Here's how the part is built. I have some questions about the finished solid (model axes, mm). A direction names the side the tool comes from. Give positions to 0.01 mm unless a question says otherwise; leave off trailing zeros. Loops run counter-clockwise (first coordinate to the right, second up) from the corner with the lowest first, then second, coordinate; pieces in that order, holes last. Notation, with made-up numbers: (78.5, 72.5) - (89.5, 72.5) arc R19 cw to (89.5, 105.5) - close; hole circle Ø5 at (20, 84.25). An arc over 180 degrees is marked (long way). Use one line per item in the form item = value.
from build123d import *

# Parameters (mm, degrees)
EXTRUDE_1_DEPTH           = 200
CUT_EXTRUDE_START         = -130
CUT_EXTRUDE_1_OUTLINE_W   = 315
CUT_EXTRUDE_1_OUTLINE_H   = 262
CUT_EXTRUDE_1_DEPTH       = 65
CUT_EXTRUDE_START_2       = 65
CUT_EXTRUDE_1_2_OUTLINE_W = 315
CUT_EXTRUDE_1_2_OUTLINE_H = 262
CUT_EXTRUDE_1_2_DEPTH     = 65
SHELL_START               = 5
SHELL_1_OUTLINE_W         = 125
SHELL_1_OUTLINE_H         = 250
SHELL_1_DEPTH             = 190
EXTRUDE_7_DEPTH           = 3
SKETCH_5_R                = 5
EXTRUDE_8_DEPTH           = 5
SKETCH_6_R                = 38
SKETCH_6_R_2              = 16
EXTRUDE_9_DEPTH           = 15
SKETCH_7_R                = 10
SKETCH_7_R_2              = 5
EXTRUDE_10_DEPTH          = 15
SKETCH_8_R                = 1.5
CUT_EXTRUDE_2_DEPTH       = 10


with BuildPart() as part:
    # 草图1 → 旋转1 (revolve)
    with BuildSketch(Plane.XY):
        with BuildLine():
            Line((0, 130), (0, -130))
            ThreePointArc((0, -130), (130, 0), (0, 130))
        make_face()
    revolve(axis=Axis((0, 130, 0), (0, -1, 0)))

    # 草图3 → 凸台-拉伸1 (add)
    with BuildSketch(Plane(origin=(0, 0, 0), x_dir=(1, 0, 0), z_dir=(0, 1, 0))):
        with BuildLine():
            Line((-120, -130), (120, -130))
            ThreePointArc((120, -130), (127.071067812, -127.071067812), (130, -120))
            Line((130, -120), (130, 120))
            ThreePointArc((130, 120), (127.071067812, 127.071067812), (120, 130))
            Line((120, 130), (-120, 130))
            ThreePointArc((-120, 130), (-127.071067812, 127.071067812), (-130, 120))
            Line((-130, 120), (-130, -120))
            ThreePointArc((-130, -120), (-127.071067812, -127.071067812), (-120, -130))
        make_face()
    extrude(amount=EXTRUDE_1_DEPTH)

    # 切除-拉伸1: read off the stored shape, not the designer's step
    # 切除-拉伸1 outline → 切除-拉伸1 (cut)
    with BuildSketch(Plane.YZ.offset(CUT_EXTRUDE_START)):
        with Locations((43.5, 0)):
            Rectangle(CUT_EXTRUDE_1_OUTLINE_W, CUT_EXTRUDE_1_OUTLINE_H)
    extrude(amount=CUT_EXTRUDE_1_DEPTH, mode=Mode.SUBTRACT)

    # Cut-Extrude 1 2 outline → Cut-Extrude 1 2 (cut)
    with BuildSketch(Plane.YZ.offset(CUT_EXTRUDE_START_2)):
        with Locations((43.5, 0)):
            Rectangle(CUT_EXTRUDE_1_2_OUTLINE_W, CUT_EXTRUDE_1_2_OUTLINE_H)
    extrude(amount=CUT_EXTRUDE_1_2_DEPTH, mode=Mode.SUBTRACT)

    # 抽壳1: read off the stored shape, not the designer's step
    # 抽壳1 outline → 抽壳1 (cut)
    with BuildSketch(Plane(origin=(0, 0, 0), x_dir=(1, 0, 0), z_dir=(0, 1, 0)).offset(SHELL_START)):
        with Locations((-2.5, 0)):
            Rectangle(SHELL_1_OUTLINE_W, SHELL_1_OUTLINE_H)
    extrude(amount=SHELL_1_DEPTH, mode=Mode.SUBTRACT)

    # Shell 1 2 outline → Shell 1 2 (revolve, cut)
    with BuildSketch(Plane.YX):
        with BuildLine():
            Line((109.658560943, 60.0000001), (0, 60.000000075))
            Line((0, 60.000000075), (0, -65.0000001))
            Line((0, -65.0000001), (106.770782459, -65.0000001))
            ThreePointArc((106.770782459, -65.0000001), (124.966656288, -2.887008165), (109.658560943, 60.0000001))
        make_face()
    revolve(axis=Axis((0, 0, 0), (1, 0, 0)), mode=Mode.SUBTRACT)

    # 草图4 → 凸台-拉伸7 (add)
    with BuildSketch(Plane.ZY.offset(65)):
        with BuildLine():
            Line((-130, 135), (-130, 0))
            Line((-130, 0), (-112.249721603, 0))
            ThreePointArc((-112.249721603, 0), (0, 112.249721603), (112.249721603, 0))
            Line((112.249721603, 0), (130, 0))
            Line((130, 0), (130, 135))
            Line((130, 135), (-130, 135))
        make_face()
    extrude(amount=-EXTRUDE_7_DEPTH)

    # 草图5 → 凸台-拉伸8 (add)
    with BuildSketch(Plane(origin=(0, 200, 0), x_dir=(1, 0, 0), z_dir=(0, 1, 0))):
        with Locations(Location((-45.093986565, 120.067321952, 0), (0, 0, 270))):
            Circle(SKETCH_5_R)
        with Locations(Location((-45.093986565, -120.067321952, 0), (0, 0, 90))):
            Circle(SKETCH_5_R)
        with Locations(Location((45.093986565, -120.067321952, 0), (0, 0, 270))):
            Circle(SKETCH_5_R)
        with Locations(Location((45.093986565, 120.067321952, 0), (0, 0, 90))):
            Circle(SKETCH_5_R)
    extrude(amount=EXTRUDE_8_DEPTH)

    # 草图6 → 凸台-拉伸9 (add)
    with BuildSketch(Plane.ZY.offset(-60)):
        with Locations(Location((0, 0, 0), (0, 0, 180))):
            Circle(SKETCH_6_R)
        Circle(SKETCH_6_R_2, mode=Mode.SUBTRACT)
    extrude(amount=EXTRUDE_9_DEPTH)

    # 草图7 → 凸台-拉伸10 (add)
    with BuildSketch(Plane.ZY.offset(-60)):
        with Locations(Location((-92.612625974, 96.844728871, 0), (0, 0, 180))):
            Circle(SKETCH_7_R)
        with Locations((-92.612625974, 96.844728871)):
            Circle(SKETCH_7_R_2, mode=Mode.SUBTRACT)
    extrude(amount=EXTRUDE_10_DEPTH)

    # 草图8 → 切除-拉伸2 (cut)
    with BuildSketch(Plane(origin=(0, 0, -130), x_dir=(-1, 0, 0), z_dir=(0, 0, -1))):
        with Locations((-26.070809392, 147.850864108)):
            Circle(SKETCH_8_R)
        with Locations((-7.111216047, 147.850864108)):
            Circle(SKETCH_8_R)
        with Locations((-26.070809392, 127.113089979)):
            Circle(SKETCH_8_R)
        with Locations((-7.111216047, 127.113089979)):
            Circle(SKETCH_8_R)
    extrude(amount=-CUT_EXTRUDE_2_DEPTH, mode=Mode.SUBTRACT)


solid = part.part
(1) Thinking about a two-plate mould opening in Z: for faces 6 (the cylindrical face through (-63.521, 112.224, -2.398)), 7 (the flat face through (49, 0, -125)), 8 (the flat face through (1, 99, -130)), which applies, pulls with the +Z half, pulls with the -Z half, needs draft (parallel to the pull), parting line crosses it, or undercut?
Geometry says:
face_6 = undercut
face_7 = needs draft
face_8 = pulls with the -Z half
(2) If we section it at D-D (z = 75): List the corners of the cut face in (x, y) for me.
Geometry says:
outline = (-65, -83.96) arc R106.18 ccw to (65, -83.96) - (65, 200) - (-65, 200) - (-65, 195) - (60, 195) - (60, -80) arc R100 cw to (-65, -75.99) - close; (-65, 83.52) - (-62, 83.52) - (-62, 135) - (-65, 135) - close
(3) If we section it at B-B (x = -26.5): List the corners of the cut face in (y, z) for me.
Geometry says:
outline = (0, -130) - (200, -130) - (200, 130) - (0, 130) - (0, 127.27) arc R127.27 ccw to (0, -127.27) - close; hole (5, -125) - (195, -125) - (195, 125) - (5, 125) - (5, 122.06) arc R122.16 ccw (long way) to (5, -122.06) - close
(4) If we section it at C-C (y = 178): List the corners of the cut face in (x, z) for me, plus the area to 3 significant figures.
Geometry says:
outline = (-65, -130) - (65, -130) - (65, 130) - (-65, 130) - (-65, 125) - (60, 125) - (60, -125) - (-65, -125) - close
area = 2,550 mm²
(5) If I drill on probe 1 along Z at (x, y) = (-42, 65); probe 2 along X at (y, z) = (60, 95); probe 3 along Y at (x, z) = (25.5, -59), over which ranges is the centre line in solid material (lowest first)?
Geometry says:
probe_1 = -130 to -125, 125 to 130
probe_2 = -65 to -62, 60 to 65
probe_3 = -113 to -107.21, 195 to 200
(6) For faces 1 (the flat face through (-50, 0, 124)), 2 (the cylindrical face through (44.874, 202.465, -115.072)), 3 (the flat face through (45, 205, 120)), 4 (the flat face through (-62, 114, -2)), 5 (the cylindrical face through (52.605, 37.096, 8.238)), which set-ups out of +Z, -Z, +X, -X, +Y, -Y let a thin tool reach every point of the face, with its end or its side?
Geometry says:
face_1 = +Z, -X, -Y
face_2 = +Y
face_3 = +Z, -Z, +X, -X, +Y
face_4 = none
face_5 = -X
(7) If we section it at A-A (z = 0): List the corners of the cut face in (x, y) for me.
Geometry says:
outline = (-65, -112.58) arc R130 ccw to (65, -112.58) - (65, 200) - (-65, 200) - (-65, 195) - (60, 195) - (60, 38) - (45, 38) - (45, 16) - (60, 16) - (60, -16) - (45, -16) - (45, -38) - (60, -38) - (60, -109.66) arc R125 cw to (-65, -106.77) - close; (-65, 112.25) - (-62, 112.25) - (-62, 135) - (-65, 135) - close
(8) For P1, Ø5.5, axis at x = 21, z = 117.5, coming from the +Y side; P2, Ø19, axis at y = 0, z = 0, coming from the -X side; P3, Ø10, axis at x = 2.5, y = -87.5, coming from the +Z side; P4, Ø4, axis at x = 7.11, y = 147.85, coming from the -Z side, each with a flat end and sliding along its axis, tell me the tip position at first contact or that it passes through.
Geometry says:
P1 = 200
P2 = 60
P3 = 100.44
P4 = -130
